```python
from build123d import *

# Parameters (mm, degrees)
SHEET_EXTRUDE_1_1_DEPTH = 30
THICKEN_1_T2            = 4
CUT_EXTRUDE_1_DEPTH     = 30
FILLET_1_R              = 1
FILLET_2_R              = 1


with BuildPart() as body_1:
    # Sheet Extrude 1: a surface, the sketch's curves swept straight by 30 mm
    with BuildLine(Plane.XY, mode=Mode.PRIVATE) as sheet_extrude_1_1_path:
        Line((12, 15), (0, 15))
        Line((0, 15), (0, 0))
        Line((0, 0), (12, 0))
    sheet_extrude_1_1 = Shell.extrude(sheet_extrude_1_1_path.wire(), (0 * SHEET_EXTRUDE_1_1_DEPTH, 0 * SHEET_EXTRUDE_1_1_DEPTH, 1 * SHEET_EXTRUDE_1_1_DEPTH))
    add(Solid.thicken(sheet_extrude_1_1, -THICKEN_1_T2))

    # 草图2 → 切除-拉伸1 (cut)
    with BuildSketch(Plane(origin=(0, 19, 0), x_dir=(1, 0, 0), z_dir=(0, 1, 0))):
        with BuildLine():
            ThreePointArc((3.46625552, -4.537501621), (4.712321266, -3.283579711), (3.458399356, -2.037513964))
            ThreePointArc((3.458399356, -2.037513964), (2.21233361, -3.291435874), (3.46625552, -4.537501621))
        make_face()
        with BuildLine():
            ThreePointArc((9.466225894, -4.518646828), (10.712291641, -3.264724918), (9.458369731, -2.018659172))
            ThreePointArc((9.458369731, -2.018659172), (8.212303985, -3.272581082), (9.466225894, -4.518646828))
        make_face()
        with BuildLine():
            ThreePointArc((3.541674691, -28.537383119), (4.787740437, -27.283461209), (3.533818527, -26.037395463))
            ThreePointArc((3.533818527, -26.037395463), (2.287752781, -27.291317373), (3.541674691, -28.537383119))
        make_face()
        with BuildLine():
            ThreePointArc((9.541645066, -28.518528326), (10.787710812, -27.264606416), (9.533788902, -26.01854067))
            ThreePointArc((9.533788902, -26.01854067), (8.287723156, -27.27246258), (9.541645066, -28.518528326))
        make_face()
    extrude(amount=-CUT_EXTRUDE_1_DEPTH, mode=Mode.SUBTRACT)

    # 圆角1
    fillet_1_edges = [body_1.edges().sort_by_distance(p)[0] for p in [
        (12, -2, 30),
        (12, 17, 30),
        (12, 17, 0),
        (12, -2, 0),
        (0, 15, 15),
        (0, 0, 15),
    ]]
    fillet(fillet_1_edges, radius=FILLET_1_R)

    # 圆角2
    fillet_2_edges = [body_1.edges().sort_by_distance(p)[0] for p in [
        (-4, -4, 15),
        (-4, 19, 15),
    ]]
    fillet(fillet_2_edges, radius=FILLET_2_R)


solid = body_1.part
```
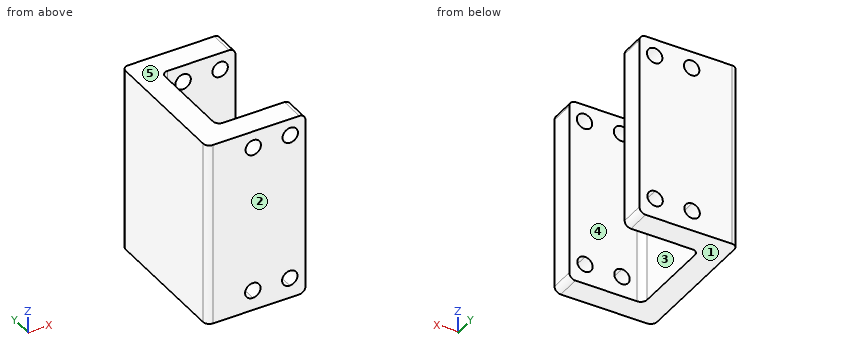
Check sheet for the modelled part. Datum: model origin and axes. Units: mm. Face numbers are marked on the shaded views. A direction names the side the tool comes from. Round coordinates to 2 decimals unless told otherwise and drop trailing zeros. Loops run counter-clockwise (first coordinate to the right, second up) from the corner with the lowest first, then second, coordinate; pieces in that order, holes last. Notation, with made-up numbers: (18, 43.5) -> (31, 43.5) arc R28 cw to (31, 82.5) -> close; hole circle Ø8 at (38.5, -37.5). An arc over 180 degrees is marked (long way). Answer in a Markdown table with one row per item.
Q1. Release check for a two-part mould opening along Y. For the marked faces 1, 2 and 3 record: released by +Y, released by -Y, zero draft, split by the parting line, or undercut.
Data:
| item | result |
|---|---|
| face 1 | zero draft |
| face 2 | released by -Y |
| face 3 | undercut |
Q2. Thickness scan on L1, parallel to Z at x = 3.25, y = -0.25; L2, parallel to Y at x = 2, z = 23; L3, parallel to X at y = 11.75, z = 7.5. Record the ranges inside material, lowest first.
Data:
| item | result |
|---|---|
| L1 | z = 0 to 2.06, 4.52 to 26.07, 28.5 to 30 |
| L2 | y = -4 to 0, 15 to 19 |
| L3 | x = -4 to 0 |
Q3. Sectioned sample at B-B on z = 10.5. Enter the section's corners in (x, y).
Data:
| item | result |
|---|---|
| outline | (-4, -3) arc R1 ccw to (-3, -4) -> (12, -4) -> (12, 0) -> (1, 0) arc R1 cw to (0, 1) -> (0, 14) arc R1 cw to (1, 15) -> (12, 15) -> (12, 19) -> (-3, 19) arc R1 ccw to (-4, 18) -> close |
Q4. Sectioned sample at A-A on x = 5.25. Enter the section's corners in (y, z).
Data:
| item | result |
|---|---|
| outline | (-4, 0) -> (0, 0) -> (0, 30) -> (-4, 30) -> close; (15, 0) -> (19, 0) -> (19, 30) -> (15, 30) -> close |
Q5. Go/stop test with flat-tipped pins: P1, Ø4, axis at x = 3.54, z = 27.29, coming from the -Y side; P2, Ø6.5, axis at y = 5, z = 13.5, coming from the +X side; P3, Ø2, axis at x = 3.54, z = 27.29, coming from the -Y side. Record where each tip stops, or that it passes through.
Data:
| item | result |
|---|---|
| P1 | stops at y = -4 |
| P2 | stops at x = 0 |
| P3 | passes through |
Q6. Sectioned sample at D-D on y = 17.5. Enter the section's corners in (x, z), then the cut area to 3 significant figures.
Data:
| item | result |
|---|---|
| outline | (-4, 0) -> (11, 0) arc R1 ccw to (12, 1) -> (12, 29) arc R1 ccw to (11, 30) -> (-4, 30) -> close; hole circle Ø2.5 at (3.46, 3.29); hole circle Ø2.5 at (3.54, 27.29); hole circle Ø2.5 at (9.46, 3.27); hole circle Ø2.5 at (9.54, 27.27) |
| area | 460 mm^2 |
Q7. Set-up check for the marked faces 4 and 5: record each of +Z, -Z, +X, -X, +Y, -Y from which the full face is reachable in a straight line by a thin tool's end or side.
Data:
| item | result |
|---|---|
| face 4 | +Z, -Z, +X |
| face 5 | +Z, +X, -X, +Y, -Y |
Q8. Sectioned sample at C-C on x = 10.25. Enter the section's corners in (y, z).
Data:
| item | result |
|---|---|
| outline | (-4, 0) -> (0, 0) -> (0, 2.3) -> (-4, 2.3) -> close; (-4, 4.24) -> (0, 4.24) -> (0, 26.24) -> (-4, 26.24) -> close; (-4, 28.3) -> (0, 28.3) -> (0, 30) -> (-4, 30) -> close; (15, 0) -> (19, 0) -> (19, 2.3) -> (15, 2.3) -> close; (15, 4.24) -> (19, 4.24) -> (19, 26.24) -> (15, 26.24) -> close; (15, 28.3) -> (19, 28.3) -> (19, 30) -> (15, 30) -> close |
